Geometry: see drawing. Coordinates: mm, zero at the bounding-box minimum. A direction names the side the tool comes from. Give positions to 0.01 mm unless a question says otherwise; leave off trailing zeros. Write each loop counter-clockwise with the first axis right and the second up, starting at its lowest first coordinate (ties: lowest second). Pieces come first, ordered by that corner, then holes. Notation, with made-up numbers: (30, -40) -> (73, -40) arc R17 cw to (73, -11) -> close; hole circle Ø10 at (42.25, -31). An arc over 180 degrees is marked (long way). Write item = value, one per line.
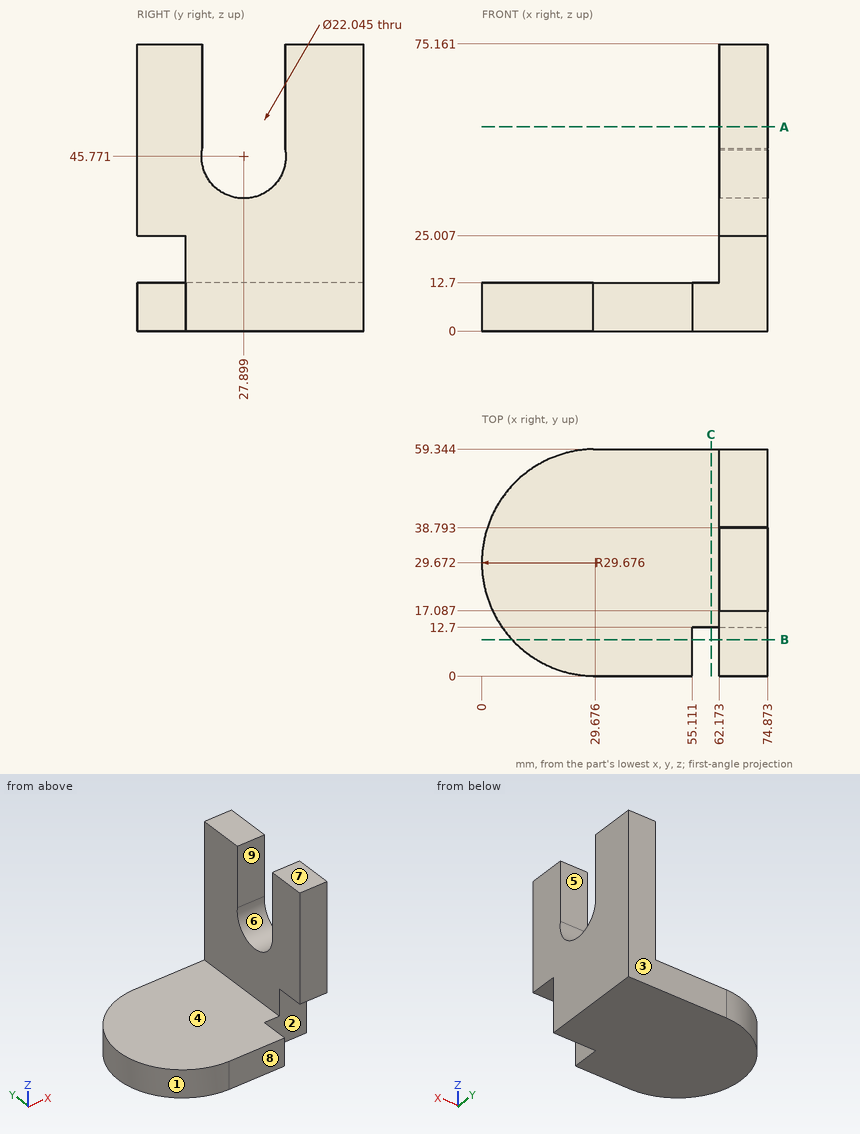
(1) Section query B-B (y = 9.5). Return loops of the section in (x, z).
Values follow:
outline = (7.91, 0) -> (55.11, 0) -> (55.11, 12.7) -> (7.91, 12.7) -> close; (62.17, 25.01) -> (74.87, 25.01) -> (74.87, 75.16) -> (62.17, 75.16) -> close
(2) Access query for the marked faces 1, 2, 3, 4 and 5. Directions: +Z, -Z, +X, -X, +Y, -Y. A direction counts if a zero-diameter tool reaches every point of the face in a straight line with its end or side. Return the directions, or none.
Values follow:
face_1 = +Z, -Z, -X
face_2 = -Z, +X, -Y
face_3 = +Z, -Z, +X, -X, +Y
face_4 = +Z, -X, +Y, -Y
face_5 = +Z, +X, -X
(3) First-contact query: pin 1 (4 mm diameter, centred on y = 47.5, z = 53, fed in from -X); pin 2 (10 mm diameter, centred on x = 68.5, y = 7.5, fed in from -Z); pin 3 (16 mm diameter, centred on x = 69.5, z = 15.5, fed in from -Y); pin 4 (5 mm diameter, centred on y = 20, z = 45, fed in from -X). Flat tips, straight axial feed; report the tip coordinate or a pass-through.
Values follow:
pin_1 = 62.17
pin_2 = 25.01
pin_3 = 12.7
pin_4 = through
(4) Section query A-A (z = 53.5). Return loops of the section in (x, y).
Values follow:
outline = (62.17, 0) -> (74.87, 0) -> (74.87, 17.09) -> (62.17, 17.09) -> close; (62.17, 38.79) -> (74.87, 38.79) -> (74.87, 59.34) -> (62.17, 59.34) -> close
(5) Section query C-C (x = 60). Return loops of the section in (y, z), plus the area to 3 significant figures.
Values follow:
outline = (12.7, 0) -> (59.34, 0) -> (59.34, 12.7) -> (12.7, 12.7) -> close
area = 592 mm2
(6) Pull-direction query (Y, two-part tool) for the marked faces 6, 7, 8 and 9; classes: pulls with the +Y half, pulls with the -Y half, needs draft (parallel to the pull), parting line crosses it, or undercut.
Values follow:
face_6 = undercut
face_7 = needs draft
face_8 = pulls with the -Y half
face_9 = undercut
(7) Material intervals for line 1 (Z direction, x = 41.5, y = 34.5); line 2 (X direction, y = 5.5, z = 52); line 3 (Y direction, x = 69.5, z = 22), sorted ascending.
Values follow:
line_1 = 0 to 12.7
line_2 = 62.17 to 74.87
line_3 = 12.7 to 59.34
